Autodesk Inventor part; units mm, degrees
ref_plane "YZ Plane" through (0, 0, 0) normal (1, 0, 0) x (0, 1, 0)
ref_plane "XZ Plane" through (0, 0, 0) normal (0, 1, 0) x (-1, 0, 0)
ref_plane "XY Plane" through (0, 0, 0) normal (0, 0, 1) x (1, 0, 0)
sketch "Sketch1" plane through (0, 0, 0) normal (0, 0, 1) x (1, 0, 0)
  line L0 (0, -25.6) -> (0, 20.6)
  line L1 (0, 3.5) -> (7.625, 3.5)
  line L2 (7.625, 3.5) -> (7.625, 14)
  line L3 (7.625, 14) -> (10.125, 14)
  line L4 (10.125, 14) -> (10.125, 1)
  line L5 (10.125, 1) -> (2, 1)
  line L6 (2, 1) -> (2, -19)
  line L7 (2, -19) -> (0, -19)
  line L8 (0, 3.5) -> (-7.625, 3.5)
  line L9 (-7.625, 3.5) -> (-7.625, 14)
  line L10 (-7.625, 14) -> (-10.125, 14)
  line L11 (-10.125, 14) -> (-10.125, 1)
  line L12 (-10.125, 1) -> (-2, 1)
  line L13 (-2, 1) -> (-2, -19)
  line L14 (-2, -19) -> (0, -19)
  line L15 (-2, 5.5) -> (2, 5.5)
  line L16 (2, 5.5) -> (2, 3.5)
  line L17 (2, 3.5) -> (-2, 3.5)
  line L18 (-2, 3.5) -> (-2, 5.5)
  point P0 (0, 0)
  point P1 (0, 5.5)
  dimension "d0" = 2.5
  dimension "d1" = 20.25
  dimension "d2" = 4
  dimension "d3" = 4
  dimension "d4" = 2
  dimension "d5" = 10.5
  dimension "d6" = 2.5
  dimension "d7" = 20
extrude "Extrusion1" add sketch "Sketch1" along normal blind 1
fillet "Fillet1" radius 1 4 edges at (-7.625, 14, 0.5) (-10.125, 14, 0.5) (7.625, 14, 0.5) (10.125, 14, 0.5)
fillet "Fillet2" radius 1 4 edges at (-2, 5.5, 0.5) (2, 5.5, 0.5) (2, 3.5, 0.5) (-2, 3.5, 0.5)
fillet "Fillet3" radius 2 4 edges at (-10.125, 1, 0.5) (10.125, 1, 0.5) (-7.625, 3.5, 0.5) (7.625, 3.5, 0.5)
properties part number "ASAP_Handle_Fixture_New2"
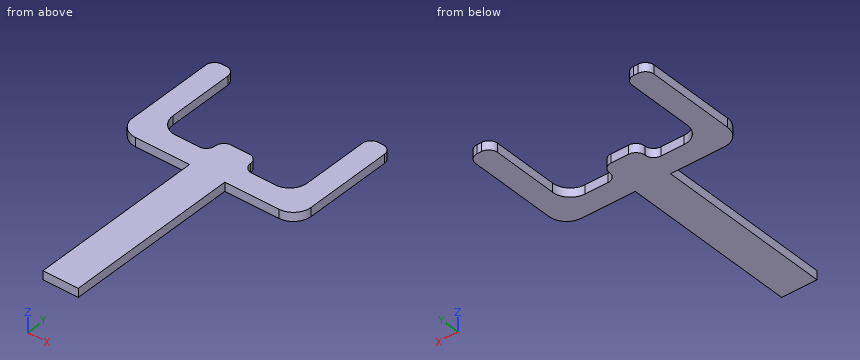
Read the model definition and answer for the solid it produces. Units are mm, in the model's axes. Coordinates: 2 decimals unless noted, no trailing zeros. Order: outer loops, then holes, each group sorted by start corner. A loop starts at its lowest first (then second) coordinate and runs counter-clockwise, first axis right, second up. Notation, with made-up numbers: (82.25, 13) - (99.25, 13) arc R15 ccw to (99.25, 34) - close; hole circle Ø1 at (76.25, -13). An arc over 180 degrees is marked (long way). Answer as a JSON object with one key per item and string values. Group by question number.
Item 1: Section D-D (y = -2) is taken. Give the vertices of the cut face in (x, z), plus the area to 3 significant figures.
Item 2: Consider probe 1 along X at (y, z) = (6, 0.85) (3 decimals); probe 2 along X at (y, z) = (-5, 0.8); probe 3 along Y at (x, z) = (-1, 0.8). Determine where each line is inside the solid, lowest interval first. Write a range as from..to.
Item 3: Flat-ended cylindrical pins translate along their axes: P1, Ø0.5, axis at y = -13, z = 0.5, coming from the -X side; P2, Ø0.5, axis at x = 4.5, z = 0.5, coming from the +Y side. Find the tip coordinate at first contact, or state that the pin passes through.
Item 4: Section A-A (y = 8) is taken. Give the vertices of the cut face in (x, z) (3 decimals), plus the area to 3 significant figures.
Item 5: Section C-C (x = 3.75) is taken. Give the vertices of the cut face in (y, z), plus the area to 3 significant figures.
Results are:
{
 "1": {"outline": "(-2, 0) - (2, 0) - (2, 1) - (-2, 1) - close", "area": "4.00 mm^2"},
 "2": {"probe 1": "x = -10.125..-7.625, 7.625..10.125", "probe 2": "x = -2..2", "probe 3": "y = -19..5.5"},
 "3": {"P1": "stops at x = -2", "P2": "stops at y = 3.5"},
 "4": {"outline": "(-10.125, 0) - (-7.625, 0) - (-7.625, 1) - (-10.125, 1) - close; (7.625, 0) - (10.125, 0) - (10.125, 1) - (7.625, 1) - close", "area": "5.00 mm^2"},
 "5": {"outline": "(1, 0) - (3.5, 0) - (3.5, 1) - (1, 1) - close", "area": "2.50 mm^2"}
}
